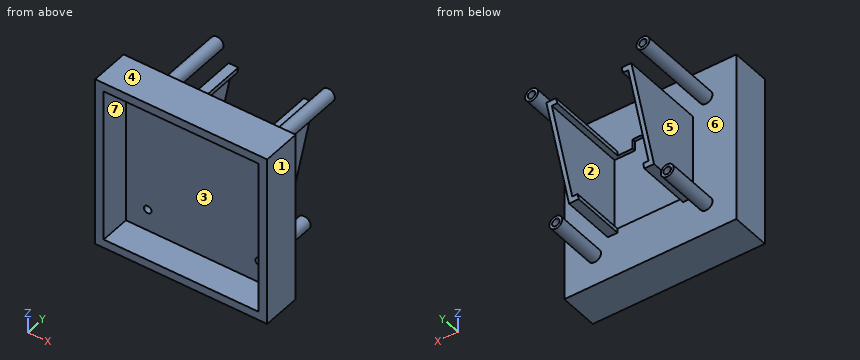
```python
from build123d import *

# Parameters (mm, degrees)
SKETCH1_W               = 80
SKETCH1_H               = 80
BOSS_EXTRUDE1_DEPTH     = 4
CUT_EXTRUDE1_DEPTH      = 1.5
BOSS_EXTRUDE2_DEPTH     = 39
SKETCH5_R               = 3
SKETCH5_R_2             = 1.75
BOSS_EXTRUDE3_DEPTH     = 40
SKETCH6_R               = 4.5
CUT_EXTRUDE2_DEPTH      = 15.39
CUT_EXTRUDE3_DEPTH      = 60.75
SKETCH9_R               = 1.75
CUT_EXTRUDE4_DEPTH      = 41
CUT_EXTRUDE4_DEPTH_BACK = 5
SKETCH10_W              = 80
SKETCH10_H              = 80
SKETCH10_W_2            = 72
SKETCH10_H_2            = 72
BOSS_EXTRUDE5_DEPTH     = 14.1


with BuildPart() as part:
    # Sketch1 → Boss-Extrude1 (new body)
    with BuildSketch(Plane(origin=(0, 0, 0), x_dir=(1, 0, 0), z_dir=(0, 1, 0))):
        Rectangle(SKETCH1_W, SKETCH1_H)
    extrude(amount=BOSS_EXTRUDE1_DEPTH)

    # Sketch2 → Cut-Extrude1 (cut)
    with BuildSketch(Plane(origin=(0, 4, 0), x_dir=(1, 0, 0), z_dir=(0, 1, 0))):
        Polygon((8.25, -17.75), (17.75, -17.75), (17.75, 17.75), (-17.75, 17.75), (-17.75, -17.75), (-8.25, -17.75), (-8.25, -22.25), (8.25, -22.25), align=None)
    extrude(amount=-CUT_EXTRUDE1_DEPTH, mode=Mode.SUBTRACT)

    # Sketch3 → Boss-Extrude2 (add)
    with BuildSketch(Plane(origin=(0, 4, 0), x_dir=(1, 0, 0), z_dir=(0, 1, 0))):
        Polygon((-19.75, 17.75), (-19.75, -17.75), (-19.75, -19.75), (-17.75, -19.75), (-15.25, -19.75), (-15.25, -17.75), (-17.75, -17.75), (-17.75, 17.75), (-15.25, 17.75), (-15.25, 19.75), (-17.75, 19.75), (-19.75, 19.75), align=None)
        Polygon((19.75, 17.75), (19.75, -17.75), (19.75, -19.75), (17.75, -19.75), (15.25, -19.75), (15.25, -17.75), (17.75, -17.75), (17.75, 17.75), (15.25, 17.75), (15.25, 19.75), (17.75, 19.75), (19.75, 19.75), align=None)
    extrude(amount=BOSS_EXTRUDE2_DEPTH)

    # Sketch5 → Boss-Extrude3 (add)
    with BuildSketch(Plane(origin=(0, 4, 0), x_dir=(1, 0, 0), z_dir=(0, 1, 0))):
        with Locations((25.9, 25.9)):
            Circle(SKETCH5_R)
        with Locations((25.9, 25.9)):
            Circle(SKETCH5_R_2, mode=Mode.SUBTRACT)
        with Locations((-25.9, 25.9)):
            Circle(SKETCH5_R)
        with Locations((-25.9, 25.9)):
            Circle(SKETCH5_R_2, mode=Mode.SUBTRACT)
        with Locations((-25.9, -25.9)):
            Circle(SKETCH5_R)
        with Locations((-25.9, -25.9)):
            Circle(SKETCH5_R_2, mode=Mode.SUBTRACT)
        with Locations((25.9, -25.9)):
            Circle(SKETCH5_R)
        with Locations((25.9, -25.9)):
            Circle(SKETCH5_R_2, mode=Mode.SUBTRACT)
    extrude(amount=BOSS_EXTRUDE3_DEPTH)

    # Sketch6 → Cut-Extrude2 (cut)
    with BuildSketch(Plane(origin=(0, 44, 0), x_dir=(1, 0, 0), z_dir=(0, 1, 0))):
        with Locations((-25.9, 25.9)):
            Circle(SKETCH6_R)
        with Locations((25.9, 25.9)):
            Circle(SKETCH6_R)
    extrude(amount=-CUT_EXTRUDE2_DEPTH, mode=Mode.SUBTRACT)

    # Sketch7 → Cut-Extrude3 (cut, through all)
    with BuildSketch(Plane.ZY.offset(19.75)):
        Polygon((-19.75, 28.61), (19.75, 43), (-19.75, 43), align=None)
    extrude(amount=-CUT_EXTRUDE3_DEPTH, mode=Mode.SUBTRACT)

    # Sketch9 → Cut-Extrude4 (cut, two sides)
    with BuildSketch(Plane(origin=(0, 4, 0), x_dir=(1, 0, 0), z_dir=(0, 1, 0))) as cut_extrude4_sk:
        with Locations((-25.9, 25.9)):
            Circle(SKETCH9_R)
        with Locations((-25.9, -25.9)):
            Circle(SKETCH9_R)
        with Locations((25.9, -25.9)):
            Circle(SKETCH9_R)
        with Locations((25.9, 25.9)):
            Circle(SKETCH9_R)
    extrude(amount=CUT_EXTRUDE4_DEPTH, mode=Mode.SUBTRACT)
    extrude(cut_extrude4_sk.sketch, amount=-CUT_EXTRUDE4_DEPTH_BACK, mode=Mode.SUBTRACT)

    # Sketch10 → Boss-Extrude5 (add)
    with BuildSketch(Plane.XZ):
        Rectangle(SKETCH10_W, SKETCH10_H)
        Rectangle(SKETCH10_W_2, SKETCH10_H_2, mode=Mode.SUBTRACT)
    extrude(amount=BOSS_EXTRUDE5_DEPTH)


solid = part.part
```
CAD build for the part. Positions are in the model's coordinates, mm. Face numbers are marked on the shaded views. A direction names the side the tool comes from. Round coordinates to 2 decimals unless told otherwise and drop trailing zeros. Order: outer loops, then holes, each group sorted by start corner. A loop starts at its lowest first (then second) coordinate and runs counter-clockwise, first axis right, second up.
Q1. Slice it at D-D (x = -25.9). Write the cut outline in (y, z), and give its area (3 significant figures).
Q2. Drop flat-ended pins along their axis: pin 1 (1.6 mm diameter, centred on y = 21, z = 19, fed in from -X); pin 2 (1.3 mm diameter, centred on x = 18, y = 27.5, fed in from +Z); pin 3 (11.5 mm diameter, centred on y = 14, z = -3, fed in from +X). Give the stop position or say it passes through.
Q3. Which spindle directions (+Z, -Z, +X, -X, +Y, -Y) get a long thin tool onto all of the face, cutting with end or side? Do the marked faces 1, 2 and 3. Say none if no direction does.
Q4. Slice it at A-A (y = 16). State how many separate pieces and enclosed holes the cut face has, and give its area (3 significant figures).
Q5. Slice it at B-B (z = -25.9). Write the cut outline in (x, y).
Q6. Wall check: L1, parallel to X at y = 2.4, z = 25.9; L2, parallel to X at y = 9.5, z = -25.9. Give the ranges that are in metal, low to high.
Q7. Slice it at C-C (y = 33.5). Write the cut outline in (x, z).
Q8. Two-plate mould, pull along Z, no slides. Class the marked faces 4, 5, 6 and 7: pulls with the +Z half, pulls with the -Z half, needs draft (parallel to the pull), parting line crosses it, or undercut.
Results below:
1. outline: (-14.1, -40) - (4, -40) - (4, -28.9) - (28.61, -28.9) - (28.61, -27.65) - (0, -27.65) - (0, -36) - (-14.1, -36) - close; (-14.1, 36) - (0, 36) - (0, 27.65) - (44, 27.65) - (44, 28.9) - (4, 28.9) - (4, 40) - (-14.1, 40) - close; (0, -24.15) - (28.61, -24.15) - (28.61, -22.9) - (4, -22.9) - (4, 22.9) - (44, 22.9) - (44, 24.15) - (0, 24.15) - close
1. area: 566 mm2
2. pin 1: stops at x = -19.75
2. pin 2: stops at z = 19.75
2. pin 3: stops at x = 19.75
3. face 1: +Z, -Z, +X, +Y, -Y
3. face 2: +Y
3. face 3: -Y
4. separate pieces: 6
4. enclosed holes: 4
4. area: 253 mm2
5. outline: (-40, -14.1) - (-36, -14.1) - (-36, 0) - (-27.65, 0) - (-27.65, 28.61) - (-28.9, 28.61) - (-28.9, 4) - (-40, 4) - close; (-24.15, 0) - (24.15, 0) - (24.15, 28.61) - (22.9, 28.61) - (22.9, 4) - (-22.9, 4) - (-22.9, 28.61) - (-24.15, 28.61) - close; (27.65, 0) - (36, 0) - (36, -14.1) - (40, -14.1) - (40, 4) - (28.9, 4) - (28.9, 28.61) - (27.65, 28.61) - close
6. L1: x = -40 to -27.65, -24.15 to 24.15, 27.65 to 40
6. L2: x = -28.9 to -27.65, -24.15 to -22.9, 22.9 to 24.15, 27.65 to 28.9
7. outline: circle Ø6 at (-25.9, 25.9); (-19.75, -6.33) - (-17.75, -6.33) - (-17.75, 17.75) - (-15.25, 17.75) - (-15.25, 19.75) - (-19.75, 19.75) - close; (15.25, 17.75) - (17.75, 17.75) - (17.75, -6.33) - (19.75, -6.33) - (19.75, 19.75) - (15.25, 19.75) - close; circle Ø6 at (25.9, 25.9); hole circle Ø3.5 at (-25.9, 25.9); hole circle Ø3.5 at (25.9, 25.9)
8. face 4: pulls with the +Z half
8. face 5: needs draft
8. face 6: undercut
8. face 7: undercut
